from build123d import *

# Parameters (mm, degrees)
SKETCH1_R           = 2.75
BOSS_EXTRUDE1_DEPTH = 18.5
CUT_EXTRUDE1_DEPTH  = 8
SKETCH3_R           = 1
CUT_EXTRUDE2_DEPTH  = 6


with BuildPart() as part:
    # Sketch1 → Boss-Extrude1 (new, symmetric)
    with BuildSketch(Plane(origin=(0, 0, 0), x_dir=(0, 0, -1), z_dir=(1, 0, 0))):
        Circle(SKETCH1_R)
    extrude(amount=BOSS_EXTRUDE1_DEPTH, both=True)

    # Sketch2 → Cut-Extrude1 (cut)
    with BuildSketch(Plane(origin=(18.5, 0, 0), x_dir=(0, 0, -1), z_dir=(1, 0, 0))):
        with BuildLine():
            Line((-1.85, 2.034698995), (-1.85, -2.034698995))
            ThreePointArc((-1.85, -2.034698995), (-2.75, 0), (-1.85, 2.034698995))
        make_face()
        with BuildLine():
            Line((1.85, 2.034698995), (1.85, -2.034698995))
            ThreePointArc((1.85, -2.034698995), (2.75, 0), (1.85, 2.034698995))
        make_face()
    cut_extrude1 = extrude(amount=-CUT_EXTRUDE1_DEPTH, mode=Mode.SUBTRACT)

    # Sketch3 → Cut-Extrude2 (cut)
    with BuildSketch(Plane(origin=(18.5, 0, 0), x_dir=(0, 0, -1), z_dir=(1, 0, 0))):
        Circle(SKETCH3_R)
    cut_extrude2 = extrude(amount=-CUT_EXTRUDE2_DEPTH, mode=Mode.SUBTRACT)

    # Mirror1: Cut-Extrude1, Cut-Extrude2 across plane
    add(cut_extrude1.mirror(Plane(origin=(0, 0, 0), x_dir=(0, 0, 1), z_dir=(1, 0, 0))), mode=Mode.SUBTRACT)
    add(cut_extrude2.mirror(Plane(origin=(0, 0, 0), x_dir=(0, 0, 1), z_dir=(1, 0, 0))), mode=Mode.SUBTRACT)


solid = part.part
The model under review builds one solid part; all positions refer to its coordinate system, in mm. A direction names the side the tool comes from. Coordinates: 2 decimals unless noted, no trailing zeros. Write each loop counter-clockwise with the first axis right and the second up, starting at its lowest first coordinate (ties: lowest second). Pieces come first, ordered by that corner, then holes. Notation, with made-up numbers: (36.25, 26.25) -> (89.25, 26.25) arc R21 cw to (89.25, 38.25) -> close; hole circle Ø2 at (-0.75, 76.5). An arc over 180 degrees is marked (long way). Answer in a Markdown table with one row per item.
1. Clearance check with flat-ended pins moving along their axes: pin 1 Ø1.2 at (x, y) = (-15, 0) entering from +Z; pin 2 Ø1 at (y, z) = (0, 0) entering from -X; pin 3 Ø1 at (y, z) = (0.5, -2.5) entering from -X. State where each tip first meets the part, or that it passes through.
Answers below:
| item | result |
|---|---|
| pin 1 | stops at z = 1.85 |
| pin 2 | stops at x = -12.5 |
| pin 3 | stops at x = -10.5 |
2. We need section B-B, the plane z = 0. State the section outline as (x, y) points, and give its area (4 significant figures).
Answers below:
| item | result |
|---|---|
| outline | (-18.5, -2.75) -> (18.5, -2.75) -> (18.5, -1) -> (12.5, -1) -> (12.5, 1) -> (18.5, 1) -> (18.5, 2.75) -> (-18.5, 2.75) -> (-18.5, 1) -> (-12.5, 1) -> (-12.5, -1) -> (-18.5, -1) -> close |
| area | 179.5 mm^2 |
3. For faces 4 (the flat face through (10.5, 0, -2.2)), 5 (the flat face through (-12.5, 0, 0)), 6 (the flat face through (-15, 0, 1.85)), 7 (the flat face through (15, 0, 1.85)), list the 3-axis set-ups (+Z, -Z, +X, -X, +Y, -Y) from which the entire face can be reached by the end or side of a thin tool; tool diameter is ignored.
Answers below:
| item | result |
|---|---|
| face 4 | -Z, +X, +Y, -Y |
| face 5 | -X |
| face 6 | +Z, -X, +Y, -Y |
| face 7 | +Z, +X, +Y, -Y |
4. Draft analysis for pull direction Z (two halves, no side actions). For faces 1 (the cylindrical face through (16, -1, 0)), 2 (the flat face through (15, 0, -1.85)), 3 (the flat face through (-10.5, 0, -2.2)), state which applies: +Z half, -Z half, draft (parallel to the pull), parting line (faces both ways), or undercut.
Answers below:
| item | result |
|---|---|
| face 1 | undercut |
| face 2 | -Z half |
| face 3 | draft |
5. Wall thickness on probe 1 along X at (y, z) = (-0.2, -0.85); probe 2 along Z at (x, y) = (12, -1.9); probe 3 along Z at (x, y) = (-2, -1.5): over which ranges is each line inside the solid? List them lowest first. Write a range as [from, to].
Answers below:
| item | result |
|---|---|
| probe 1 | x = [-12.5, 12.5] |
| probe 2 | z = [-1.85, 1.85] |
| probe 3 | z = [-2.3, 2.3] |
6. We need section D-D, the plane y = 0. State the section outline as (x, z) points.
Answers below:
| item | result |
|---|---|
| outline | (-18.5, -1.85) -> (-10.5, -1.85) -> (-10.5, -2.75) -> (10.5, -2.75) -> (10.5, -1.85) -> (18.5, -1.85) -> (18.5, -1) -> (12.5, -1) -> (12.5, 1) -> (18.5, 1) -> (18.5, 1.85) -> (10.5, 1.85) -> (10.5, 2.75) -> (-10.5, 2.75) -> (-10.5, 1.85) -> (-18.5, 1.85) -> (-18.5, 1) -> (-12.5, 1) -> (-12.5, -1) -> (-18.5, -1) -> close |
7. We need section C-C, the plane x = -8. State the section outline as (y, z) points, and give its area (3 significant figures).
Answers below:
| item | result |
|---|---|
| outline | circle Ø5.5 at (0, 0) |
| area | 23.8 mm^2 |
8. We need section A-A, the plane y = 1.65. State the section outline as (x, z) points.
Answers below:
| item | result |
|---|---|
| outline | (-18.5, -1.85) -> (-10.5, -1.85) -> (-10.5, -2.2) -> (10.5, -2.2) -> (10.5, -1.85) -> (18.5, -1.85) -> (18.5, 1.85) -> (10.5, 1.85) -> (10.5, 2.2) -> (-10.5, 2.2) -> (-10.5, 1.85) -> (-18.5, 1.85) -> close |
